Check sheet for the modelled part. Datum: model origin and axes. Units: mm. Round coordinates to 2 decimals unless told otherwise and drop trailing zeros. Loops run counter-clockwise (first coordinate to the right, second up) from the corner with the lowest first, then second, coordinate; pieces in that order, holes last. Notation, with made-up numbers: M 86.5,21.5 L 91.5,21.5 A23 cw 91.5,29.5 Z; hole C 74,48.5 d6. An arc over 180 degrees is marked long. One line per question, with ' | ' between items. Start each with the question number.
(1) Thickness scan on probe 1 along Z at (x, y) = (0, -0.5); probe 2 along X at (y, z) = (1, 75); probe 3 along X at (y, z) = (0, -20). Record the ranges inside material, lowest first. Write a range as [from, to].
(2) Section check C-C (y = 1.75). Count the separate pieces of the cut face and the enclosed holes in it, and give its area (3 significant figures).
(3) Go/stop test with flat-tipped pins: P1, Ø6.5, axis at x = 0, z = -75, coming from the -Y side (3 decimals); P2, Ø2, axis at x = -81.5, y = -1.5, coming from the +Z side (3 decimals); P3, Ø2, axis at x = -80, y = 2, coming from the -Z side; P4, Ø3, axis at x = -53.5, y = -1.5, coming from the -Z side. Record where each tip stops, or that it passes through.
(4) Section check D-D (x = -41.5). Record the boundary of the cut face in (y, z) (3 decimals), and give its area (3 significant figures).
(5) Section check B-B (x = -100). Record the boundary of the cut face in (y, z) (3 decimals), and give its area (3 significant figures).
(6) Section check A-A (z = 0). Record the boundary of the cut face in (x, y) (3 decimals), and give its area (3 significant figures).
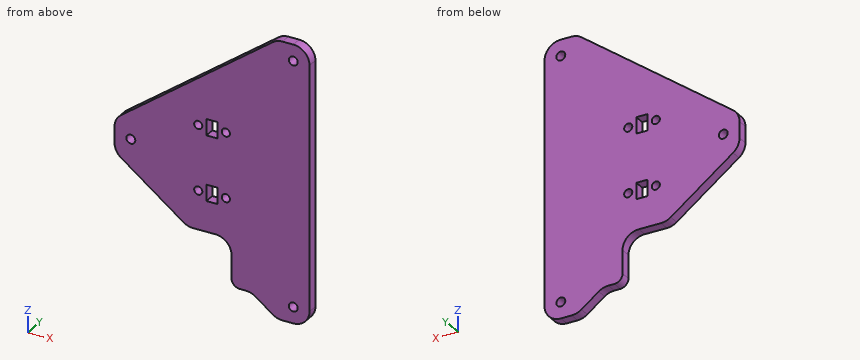
Autodesk Inventor part; units mm, degrees
ref_plane "YZ Plane" through (0, 0, 0) normal (1, 0, 0) x (0, 1, 0)
ref_plane "XZ Plane" through (0, 0, 0) normal (0, 1, 0) x (-1, 0, 0)
ref_plane "XY Plane" through (0, 0, 0) normal (0, 0, 1) x (1, 0, 0)
sketch "Sketch1" plane through (0, 0, 0) normal (0, 1, 0) x (-1, 0, 0)
  line L0 (10, -85) -> (110, -10)
  line L1 (110, -10) -> (110, 10)
  line L2 (110, 10) -> (10, 85)
  line L3 (10, 85) -> (-10, 85)
  line L4 (-10, 85) -> (-10, -85)
  line L5 (-10, -85) -> (10, -85)
  point P0 (0, 0)
  point P1 (100, 0)
  point P2 (0, -75)
  point P3 (0, 75)
  point P4 (-10, 0)
  point P5 (110, 0)
  dimension "d0" = 170
  dimension "d1" = 100
  dimension "d2" = 150
  dimension "d3" = 75
  dimension "d4" = 10
  dimension "d5" = 10
  dimension "d6" = 36.87
  dimension "d7" = 20
  dimension "d8" = 20
extrude "Extrusion1" add sketch "Sketch1" along normal mid plane 6.35
fillet "Fillet1" radius 10 6 edges at (-10, 0, 85) (10, 0, 85) (10, 0, -85) (-10, 0, -85) (-110, 0, -10) (-110, 0, 10)
sketch "Sketch2" plane through (0, 3.175, 0) normal (0, 1, 0) x (1, 0, 0)
  arc A0 (0, -85) -> (10, -75) centre (0, -75) ccw
  arc A1 (10, 75) -> (0, 85) centre (0, 75) ccw
  line L0 (-110, 5) -> (-110, -5)
  point P0 (0, 0)
  point P1 (-100, 0)
  dimension "d12" = 10
hole "Hole1" at (-100, 3.175, 0) at (0, 3.175, -75) at (0, 3.175, 75) direction (0, -1, 0) diameter 5.5 depth 7.6 tip angle 118
sketch "Sketch3" plane through (0, 3.175, 0) normal (0, 1, 0) x (1, 0, 0)
  circle A0 centre (-100, 0) radius 2.75
  line L0 (-65, 43.75) -> (-38, 43.75)
  line L1 (-38, 43.75) -> (-38, 64)
  line L2 (-38, 64) -> (-65, 43.75)
  line L3 (-12.6667, 83) -> (-106, 13)
  point P0 (0, 0)
  dimension "d20" = 35
  dimension "d21" = 27
extrude "Extrusion2" cut sketch "Sketch3" against normal blind 10 contours L2 L1 L0
sketch "Sketch6" plane through (0, 3.175, 0) normal (0, 1, 0) x (1, 0, 0)
  line L0 (-38, 43.75) -> (-38, 64)
  line L1 (-38, 64) -> (-38, 73)
  line L2 (-38, 73) -> (-26, 73)
  line L3 (-38, 64) -> (-12.6667, 83)
  point P0 (0, 0)
  dimension "d41" = 9
extrude "Extrusion4" add sketch "Sketch6" against normal up to surface (6.35 mm away)
fillet "Fillet2" radius 10 3 edges at (-65, 0, -43.75) (-38, 0, -43.75) (-26, 0, -73)
fillet "Fillet2" radius 5 1 edges at (-38, 0, -73)
sketch "Sketch4" plane through (0, -3.175, 0) normal (0, -1, 0) x (1, 0, 0)
  line L0 (-58.5, -20) -> (-41.5, -20)
  line L1 (0, 0) -> (-6.0642, 0)
  point P0 (-50, -20)
  point P1 (-58.5, 20)
  point P2 (-41.5, 20)
  point P3 (-50, 20)
  dimension "d25" = 50
  dimension "d26" = 17
  dimension "d27" = 20
hole "Hole2" at (-58.5, -3.175, -20) at (-41.5, -3.175, -20) at (-41.5, -3.175, 20) at (-58.5, -3.175, 20) at (-50, -3.175, -20) at (-50, -3.175, 20) direction (0, 1, 0) diameter 5 end through all
sketch "Sketch5" plane through (0, 3.175, 0) normal (0, 1, 0) x (1, 0, 0)
  line L0 (-38, 68) -> (-38, 53.75)
  line L1 (-48, 43.75) -> (-61.6667, 43.75)
  line L2 (-67.6667, 41.75) -> (-106, 13)
  arc A0 (-106, 13) -> (-110, 5) centre (-100, 5) ccw
  line L3 (-110, 5) -> (-110, -5)
  arc A1 (-110, -5) -> (-106, -13) centre (-100, -5) ccw
  line L4 (-106, -13) -> (-12.6667, -83)
  arc A2 (-12.6667, -83) -> (-6.6667, -85) centre (-6.6667, -75) ccw
  line L5 (-6.6667, -85) -> (0, -85)
  arc A3 (0, -85) -> (10, -75) centre (0, -75) ccw
  line L6 (10, -75) -> (10, 75)
  arc A4 (10, 75) -> (0, 85) centre (0, 75) ccw
  line L7 (0, 85) -> (-6.6667, 85)
  arc A5 (-6.6667, 85) -> (-12.6667, 83) centre (-6.6667, 75) ccw
  line L8 (-12.6667, 83) -> (-23.3333, 75)
  circle A6 centre (0, 75) radius 2.75
  circle A7 centre (-100, 0) radius 2.75
  circle A8 centre (0, -75) radius 2.75
  line L9 (-53.5, 25) -> (-46.5, 25)
  line L10 (-46.5, 25) -> (-46.5, 15)
  line L11 (-46.5, 15) -> (-53.5, 15)
  line L12 (-53.5, 15) -> (-53.5, 25)
  line L13 (-53.5, 25) -> (-46.5, 15) construction
  line L14 (-46.5, 25) -> (-53.5, 15) construction
  line L15 (-53.5, -15) -> (-46.5, -15)
  line L16 (-46.5, -15) -> (-46.5, -25)
  line L17 (-46.5, -25) -> (-53.5, -25)
  line L18 (-53.5, -25) -> (-53.5, -15)
  line L19 (-53.5, -15) -> (-46.5, -25) construction
  line L20 (-46.5, -15) -> (-53.5, -25) construction
  line L21 (-29.3333, 73) -> (-33, 73)
  arc A9 (-61.6667, 43.75) -> (-67.6667, 41.75) centre (-61.6667, 33.75) ccw
  arc A10 (-48, 43.75) -> (-38, 53.75) centre (-48, 53.75) ccw
  arc A11 (-33, 73) -> (-38, 68) centre (-33, 68) ccw
  arc A12 (-29.3333, 73) -> (-23.3333, 75) centre (-29.3333, 83) ccw
  point P0 (0, 0)
  point P1 (-50, 20)
  point P2 (-50, -20)
  dimension "d35" = 7
  dimension "d36" = 10
  dimension "d37" = 7
  dimension "d38" = 10
extrude "Extrusion3" cut sketch "Sketch5" against normal blind 10 contours L9 L10 L11 L12 | L15 L16 L17 L18
properties part number "Y_Axis_Carriage_Plate_LM3039" material "Acetal Resin, Black"
The answers:
1) probe 1: [-85, -77.75], [-72.25, 72.25], [77.75, 85] | probe 2: [-23.33, -2.75], [2.75, 10] | probe 3: [-96.67, -61], [-56, -53.5], [-46.5, -44], [-39, 10]
2) separate pieces: 1 | enclosed holes: 9 | area: 12,400 mm²
3) P1: y = -3.175 | P2: z = 32.125 | P3: z = -33.25 | P4: z = -43.75
4) outline: M -3.175,-46.151 L 3.175,-46.151 L 3.175,-22.5 L -3.175,-22.5 Z; M -3.175,-17.5 L 3.175,-17.5 L 3.175,17.5 L -3.175,17.5 Z; M -3.175,22.5 L 3.175,22.5 L 3.175,61.375 L -3.175,61.375 Z | area: 619 mm²
5) outline: M -3.175,-17.5 L 3.175,-17.5 L 3.175,-2.75 L -3.175,-2.75 Z; M -3.175,2.75 L 3.175,2.75 L 3.175,17.5 L -3.175,17.5 Z | area: 187 mm²
6) outline: M -110,-3.175 L -102.75,-3.175 L -102.75,3.175 L -110,3.175 Z; M -97.25,-3.175 L 10,-3.175 L 10,3.175 L -97.25,3.175 Z | area: 727 mm²
